Source: CAD feature listing. Evaluate the final solid. Frame: model axes, mm. A direction names the side the tool comes from. Coordinates: 2 decimals unless noted, no trailing zeros. Order: outer loops, then holes, each group sorted by start corner. A loop starts at its lowest first (then second) coordinate and runs counter-clockwise, first axis right, second up. Notation, with made-up numbers: (-13.5, -33.5) -> (26.5, -33.5) arc R14 cw to (26.5, -26.5) -> close; hole circle Ø5 at (77.25, 57.5). An arc over 180 degrees is marked (long way). Write item = value, one per line. Start each with the question number.
Item 1: Ray query, line 1 along Z through (x, y) = (-1.5, -108); line 2 along X through (y, z) = (-12.7, -3); line 3 along X through (y, z) = (-152.4, 1.5). Return the intervals inside material, ascending. Write a range as [from, to].
Item 2: Contact query for flat-ended pins moving along their axis: pin 1 (7.5 mm diameter, centred on x = -3.67, y = -12.7, fed in from +Z); pin 2 (5 mm diameter, centred on x = -54.47, y = -12.7, fed in from -Z); pin 3 (4 mm diameter, centred on x = 61.5, y = -13.5, fed in from +Z); pin 4 (1.5 mm diameter, centred on y = -63, z = 44.5, fed in from +X). Output: stop coordinate, or through.
Item 3: Section query B-B (z = 14). Output: boundary loops of the cut face in (x, y), then the cut area to 3 significant figures.
Item 4: Section query D-D (x = -10.5). Output: boundary loops of the cut face in (y, z), then the cut area to 3 significant figures.
Item 5: Mould query, pull axis Y, two halves, no side actions, for faces 3 (the cylindrical face through (-3.26, -155.55, 0.09)), 4 (the flat face through (-5, -94, 6.35)), 5 (the flat face through (26, -190.5, 5)). Classes: released by +Y, released by -Y, zero draft, split by the parting line, or undercut.
Item 6: Set-up query: faces 1 (the cylindrical face through (-5.377, -78.877, 0.089)), 2 (the flat face through (60, -13, 17.348)). Return all of +Z, -Z, +X, -X, +Y, -Y with unobstructed straight access to the full face (end or side cutting, diameter ignored); none if empty.
```python
from build123d import *

# Parameters (mm, degrees)
F1_DEPTH = 190.5
F3_D     = 6.35
F5_DEPTH = 10.9982
F7_DEPTH = 21.9964


with BuildPart() as f1:
    # F0 (on Front) → F1 (new body)
    with BuildSketch(Plane.XZ):
        with BuildLine():
            ThreePointArc((100.319202, 10.474446), (100.319202, 2.225554), (93.175452, 6.35))
            Line((93.175452, 6.35), (-93.175452, 6.35))
            Line((-93.175452, 6.35), (-105.2703, 6.35))
            Line((-105.2703, 6.35), (-105.2703, -6.35))
            Line((-105.2703, -6.35), (105.2703, -6.35))
            Line((105.2703, -6.35), (140.6906, 54.999759))
            Line((140.6906, 54.999759), (129.692077, 61.349759))
            Line((129.692077, 61.349759), (100.319202, 10.474446))
        make_face()
    extrude(amount=F1_DEPTH)

    # F3 (through all)
    with Locations(Plane(origin=(0, 0, -6.35), x_dir=(1, 0, 0), z_dir=(0, 0, -1))):
        with Locations((-3.6703, 152.4), (-3.6703, 76.2), (-3.6703, 12.7), (-54.4703, 12.7)):
            Hole(F3_D / 2)

    # F4 (on face) → F5 (join)
    with BuildSketch(Plane.XY.offset(6.35)):
        with BuildLine():
            ThreePointArc((59.8297, -6.35), (55.339572, -17.190128), (66.1797, -12.7))
            ThreePointArc((66.1797, -12.7), (64.319828, -8.209872), (59.8297, -6.35))
        make_face()
    extrude(amount=F5_DEPTH)

    # F6 (on face) → F7 (join)
    with BuildSketch(Plane(origin=(70.703833, 0, -40.820877), x_dir=(0, -1, 0), z_dir=(-0.866025, 0, 0.5))):
        with BuildLine():
            ThreePointArc((6.35, 92.576489), (12.7, 86.226489), (19.05, 92.576489))
            ThreePointArc((19.05, 92.576489), (12.7, 98.926489), (6.35, 92.576489))
        make_face()
    extrude(amount=F7_DEPTH)


solid = f1.part
```
Computed:
q1.line_1 = [-6.35, 6.35]
q1.line_2 = [-105.27, -57.65], [-51.3, -6.85], [-0.5, 107.2]
q1.line_3 = [-105.27, -6.85], [-0.5, 109.8]
q2.pin_1 = 6.35
q2.pin_2 = through
q2.pin_3 = 17.35
q2.pin_4 = 135.06
q3.outline = circle Ø12.7 at (59.83, -12.7); (102.35, -190.5) -> (117.02, -190.5) -> (117.02, 0) -> (102.35, 0) -> close
q3.area = 2,920 mm^2
q4.outline = (-190.5, -6.35) -> (0, -6.35) -> (0, 6.35) -> (-190.5, 6.35) -> close
q4.area = 2,420 mm^2
q5.face_3 = undercut
q5.face_4 = zero draft
q5.face_5 = released by -Y
q6.face_1 = +Z, -Z
q6.face_2 = +Z, -X, +Y, -Y
